from build123d import *

# Parameters (mm, degrees)
SKETCH1_W           = 22.5
SKETCH1_H           = 65.96
BOSS_EXTRUDE1_DEPTH = 35
SKETCH2_W           = 15
SKETCH2_H           = 15.96
CUT_EXTRUDE1_DEPTH  = 35
SKETCH4_R           = 1.5
CUT_EXTRUDE2_DEPTH  = 35
SKETCH5_R           = 2.65
CUT_EXTRUDE3_DEPTH  = 2
CUT_EXTRUDE4_DEPTH  = 2.17
CUT_EXTRUDE5_DEPTH  = 27.17
FILLET1_R           = 8
FILLET2_R           = 5


with BuildPart() as part:
    # Sketch1 → Boss-Extrude1 (new body)
    with BuildSketch(Plane(origin=(0, 0, 0), x_dir=(1, 0, 0), z_dir=(0, 1, 0))):
        with Locations((0, 17.02)):
            Rectangle(SKETCH1_W, SKETCH1_H)
    extrude(amount=BOSS_EXTRUDE1_DEPTH)

    # Sketch2 → Cut-Extrude1 (cut)
    with BuildSketch(Plane(origin=(0, 35, 0), x_dir=(1, 0, 0), z_dir=(0, 1, 0))):
        with Locations((0, -7.98)):
            Rectangle(SKETCH2_W, SKETCH2_H)
    extrude(amount=-CUT_EXTRUDE1_DEPTH, mode=Mode.SUBTRACT)

    # Sketch4 → Cut-Extrude2 (cut)
    with BuildSketch(Plane.ZY.offset(11.25)):
        with Locations((12.915476268, 17.5)):
            Circle(SKETCH4_R)
    extrude(amount=-CUT_EXTRUDE2_DEPTH, mode=Mode.SUBTRACT)

    # Sketch5 → Cut-Extrude3 (cut)
    with BuildSketch(Plane.ZY.offset(11.25)):
        with Locations((12.915476268, 17.5)):
            Circle(SKETCH5_R)
    extrude(amount=-CUT_EXTRUDE3_DEPTH, mode=Mode.SUBTRACT)

    # Sketch6 → Cut-Extrude4 (cut)
    with BuildSketch(Plane(origin=(11.25, 0, 0), x_dir=(0, 0, -1), z_dir=(1, 0, 0))):
        Polygon((-13.021785536, 13.863620316), (-9.961785536, 15.630312139), (-9.961785536, 19.163695787), (-13.021785536, 20.930387611), (-16.081785536, 19.163695787), (-16.081785536, 15.630312139), align=None)
    extrude(amount=-CUT_EXTRUDE4_DEPTH, mode=Mode.SUBTRACT)

    # Sketch7 → Cut-Extrude5 (cut)
    with BuildSketch(Plane(origin=(11.25, 0, 0), x_dir=(0, 0, -1), z_dir=(1, 0, 0))):
        Polygon((-15.96, 10), (-15.96, 0), (71.192312273, 0), (70.711592722, 35), (-15.96, 35), (-15.96, 25), (54.137148325, 25), (54.137148325, 10), align=None)
    extrude(amount=-CUT_EXTRUDE5_DEPTH, mode=Mode.SUBTRACT)

    # Fillet1
    fillet1_edges = [part.edges().sort_by_distance(p)[0] for p in [
        (9.375, 10, 15.96),
        (-9.375, 10, 15.96),
    ]]
    fillet(fillet1_edges, radius=FILLET1_R)

    # Fillet2
    fillet2_edges = [part.edges().sort_by_distance(p)[0] for p in [
        (11.25, 17.5, -50),
        (-11.25, 17.5, -50),
        (0, 10, -50),
        (0, 25, -50),
    ]]
    fillet(fillet2_edges, radius=FILLET2_R)


solid = part.part
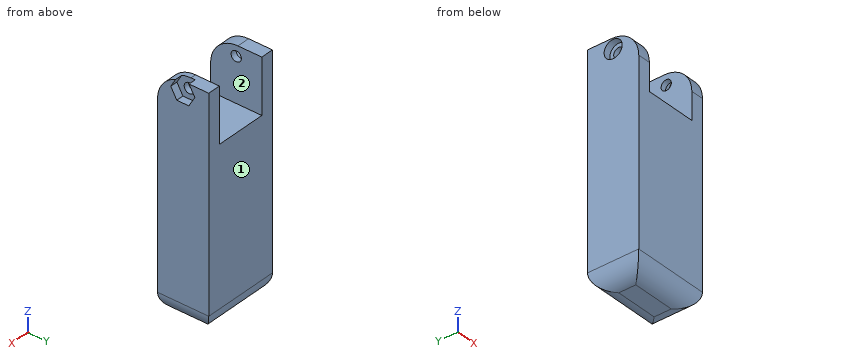
Geometry: final body of the model. Coordinates: model frame, mm. Face numbers are marked on the shaded views. A direction names the side the tool comes from. Round coordinates to 2 decimals unless told otherwise and drop trailing zeros. Loops run counter-clockwise (first coordinate to the right, second up) from the corner with the lowest first, then second, coordinate; pieces in that order, holes last. Notation, with made-up numbers: M 31,-18.75 L 67,-18.75 A23 cw 67,3.25 Z; hole C -29.5,6.5 d2. An arc over 180 degrees is marked long. One line per question, with ' | ' between items.
(1) Access query for the marked faces 1 and 2. Directions: +Z, -Z, +X, -X, +Y, -Y. A direction counts if a zero-diameter tool reaches every point of the face in a straight line with its end or side. Return the directions, or none.
Check result:
face 1: +Z, -Z, +X, -X, +Y | face 2: +Z, +Y, -Y
(2) Contact query for flat-ended pins moving along their axis: P1, Ø1.7, axis at x = 10.5, y = 18, coming from the +Z side; P2, Ø5, axis at y = 17.5, z = 12.92, coming from the +X side; P3, Ø6, axis at x = 2.5, y = 20, coming from the +Z side. Output: stop coordinate, or through.
Check result:
P1: stops at z = 9.96 | P2: stops at x = 9.08 | P3: stops at z = 0
(3) Material intervals for line 1 along X through (y, z) = (21.5, 10.5); line 2 along Z through (x, y) = (1.5, 15); line 3 along Z through (x, y) = (8.5, 17), sorted ascending. Write a range as from..to.
Check result:
line 1: x = -11.25..-7.5, 7.5..11.25 | line 2: z = -50..0 | line 3: z = -49.47..11.5, 14.33..15.9
(4) Cut plane B-B on x = -5. Return the cut outline in (y, z).
Check result:
outline: M 10,-45 A5 ccw 15,-50 L 20,-50 A5 ccw 25,-45 L 25,0 L 10,0 Z
(5) Cut plane A-A on z = 3.5. Return the cut outline in (x, y).
Check result:
outline: M -11.25,10 L -7.5,10 L -7.5,25 L -11.25,25 Z; M 7.5,10 L 11.25,10 L 11.25,25 L 7.5,25 Z
